```python
from build123d import *

# Parameters (mm, degrees)
F1_DEPTH = 5.715
F2_R     = 1.660999
F2_R_2   = 1.1938
F3_DEPTH = 19.812


with BuildPart() as f1:
    # F0 (on Front) → F1 (new body)
    with BuildSketch(Plane.XZ):
        with BuildLine():
            Line((-24.755399, 3.174997), (-52.048653, 3.156867))
            ThreePointArc((-52.048653, 3.156867), (-55.557965, 0.169667), (-52.387502, -3.175))
            Line((-52.387502, -3.175), (-24.751181, -3.175))
            ThreePointArc((-24.751181, -3.175), (-21.576181, 0), (-24.751181, 3.175))
            ThreePointArc((-24.751181, 3.175), (-24.75329, 3.174999), (-24.755399, 3.174997))
        make_face()
    extrude(amount=F1_DEPTH)

    # F2 (on face) → F3 (join)
    with BuildSketch(Plane.XZ.offset(5.715)):
        with Locations((-52.817982, 0)):
            Circle(F2_R)
        with Locations((-42.743627, 0)):
            Circle(F2_R_2)
    extrude(amount=F3_DEPTH)


solid = f1.part
```
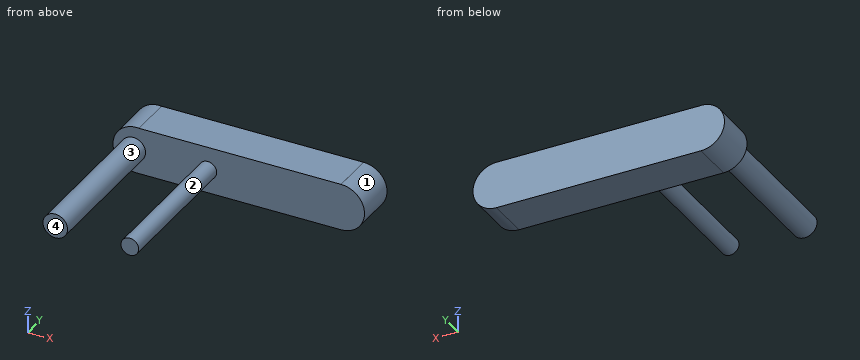
Model file for the job. Use its own axes, mm. Face numbers are marked on the shaded views. Coordinates: 2 decimals unless noted, no trailing zeros. Loops run counter-clockwise (first coordinate to the right, second up) from the corner with the lowest first, then second, coordinate; pieces in that order, holes last. Notation, with made-up numbers: M 3,-6.75 L 52,-6.75 A22 cw 52,2.25 Z; hole C 56,9 d11. An arc over 180 degrees is marked long. Use CSV: the item, a comma, the result in double quotes. Start each with the question number.
1. Two-plate mould, pull along X, no slides. Class the marked faces 1, 2, 3 and 4: pulls with the +X half, pulls with the -X half, needs draft (parallel to the pull), parting line crosses it, or undercut.
2. Band-saw the part on A-A, the plane z = 0. List the corners of the cut face in (x, y) (1 decimal).
3. Band-saw the part on D-D, the plane x = -42.5. List the corners of the cut face in (y, z) (3 decimals).
4. Probe probe 1 along Y at (x, z) = (-24, 0.5) (3 decimals); probe 2 along Z at (x, y) = (-39, -4) (3 decimals); probe 3 along X at (y, z) = (-17, 0.75). List the from-to ranges inside material, lowest first. Write a range as [from, to].
5. Flat gauge pins, fed straight in: pin 1 (2 mm diameter, centred on y = -19, z = -1, fed in from +X); pin 2 (1.9 mm diameter, centred on x = -40, z = -1.5, fed in from -Y) (3 decimals); pin 3 (8 mm diameter, centred on x = -39, y = -9.5, fed in from +Z). Where does each tip first touch, or does it go through?
6. Band-saw the part on B-B, the plane y = -19.25. List the corners of the cut face in (x, z).
Entries:
1,face 1,"pulls with the +X half"
1,face 2,"undercut"
1,face 3,"undercut"
1,face 4,"needs draft"
2,outline,"M -55.6,-5.7 L -54.5,-5.7 L -54.5,-25.5 L -51.2,-25.5 L -51.2,-5.7 L -43.9,-5.7 L -43.9,-25.5 L -41.5,-25.5 L -41.5,-5.7 L -21.6,-5.7 L -21.6,0 L -55.6,0 Z"
3,outline,"M -25.527,-1.169 L -5.715,-1.169 L -5.715,-3.175 L 0,-3.175 L 0,3.163 L -5.715,3.163 L -5.715,1.169 L -25.527,1.169 Z"
4,probe 1,"y = [-5.715, 0]"
4,probe 2,"z = [-3.175, 3.166]"
4,probe 3,"x = [-54.3, -51.34], [-43.67, -41.81]"
5,pin 1,"stops at x = -41.55"
5,pin 2,"stops at y = -5.715"
5,pin 3,"stops at z = 3.17"
6,outline,"C -52.82,0 d3.32; C -42.74,0 d2.39"
